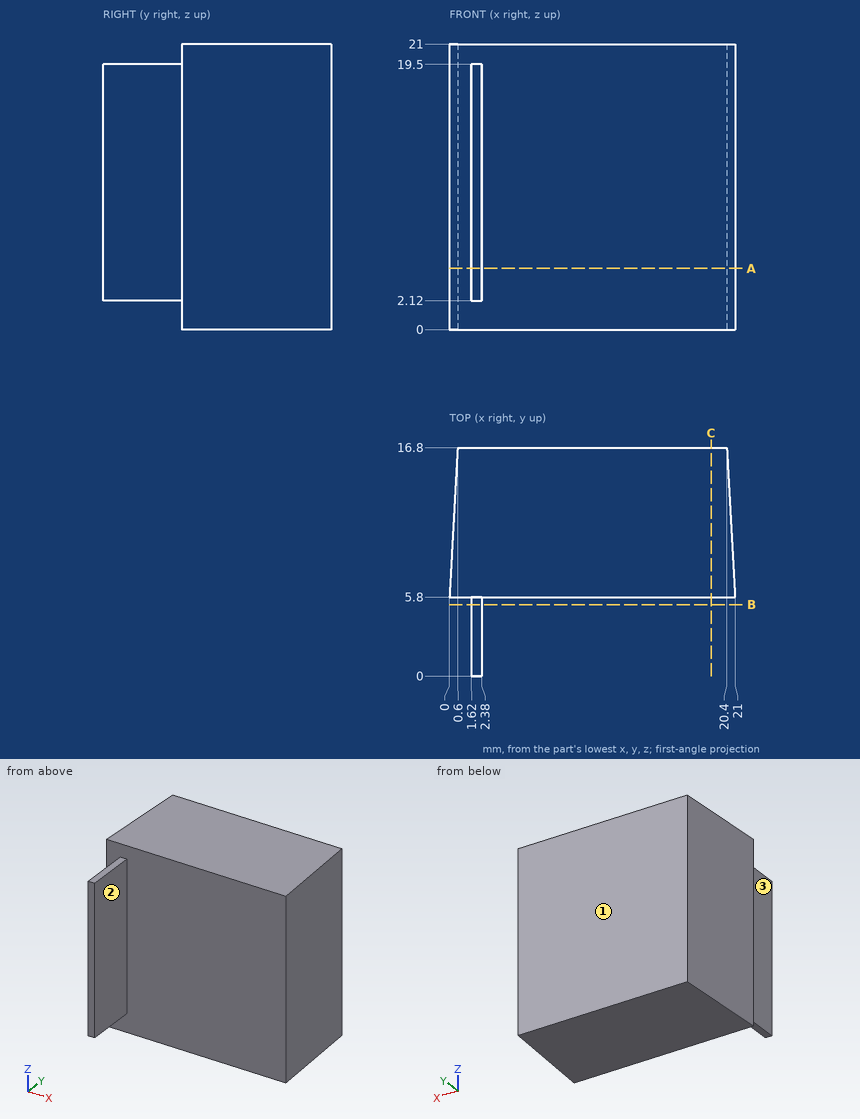
Geometry: see drawing. Coordinates: mm, zero at the bounding-box minimum. A direction names the side the tool comes from. Give positions to 0.01 mm unless a question says otherwise; leave off trailing zeros. Loops run counter-clockwise (first coordinate to the right, second up) from the corner with the lowest first, then second, coordinate; pieces in that order, holes last. Notation, with made-up numbers: (-34, 29.25) - (0, 29.25) arc R17 ccw to (0, 36.25) - close; hole circle Ø11 at (-31, 49.25). An arc over 180 degrees is marked (long way). Use CSV: the item, a comma, the result in double quotes. Start each with the question number.
Item 1: Line query: line 1 (X direction, y = 2.75, z = 8.5); line 2 (Y direction, x = 6.5, z = 8.75); line 3 (X direction, y = 14, z = 4.75). Output: solid intervals per line, ascending.
Item 2: Reachability of the marked faces 1, 2 and 3 from +Z, -Z, +X, -X, +Y, -Y: full face, straight path, thin tool, end or side. Return the list, or none.
Item 3: Section C-C on x = 19.25. Return loops of the section in (y, z).
Item 4: Contact query for flat-ended pins moving along their axis: P1, Ø0.6, axis at x = 2, y = 3.5, coming from the -Z side; P2, Ø1.7, axis at y = 2, z = 8.5, coming from the -X side; P3, Ø6.5, axis at x = 15.5, z = 5.5, coming from the -Y side. Output: stop coordinate, or through.
Item 5: Section A-A on z = 4.5. Return loops of the section in (x, y), then the cut area to 3 significant figures.
Item 6: Section B-B on y = 5.25. Return loops of the section in (x, z), then the cut area to 3 significant figures.
Ans:
1,line 1,"x = 1.62 to 2.38"
1,line 2,"y = 5.8 to 16.8"
1,line 3,"x = 0.45 to 20.55"
2,face 1,"+Z, -Z, +X, -X, +Y"
2,face 2,"+Z, -Z, +X, -Y"
2,face 3,"+Z, -Z, -X, -Y"
3,outline,"(5.8, 0) - (16.8, 0) - (16.8, 21) - (5.8, 21) - close"
4,P1,"stops at z = 2.12"
4,P2,"stops at x = 1.62"
4,P3,"stops at y = 5.8"
5,outline,"(0, 5.8) - (1.62, 5.8) - (1.62, 0) - (2.38, 0) - (2.38, 5.8) - (21, 5.8) - (20.4, 16.8) - (0.6, 16.8) - close"
5,area,"229 mm2"
6,outline,"(1.62, 2.12) - (2.38, 2.12) - (2.38, 19.5) - (1.62, 19.5) - close"
6,area,"13.2 mm2"
